```python
from build123d import *

# Parameters (mm, degrees)
SKETCH1_W           = 31
SKETCH1_H           = 15
BOSS_EXTRUDE1_DEPTH = 5
SKETCH2_W           = 15
SKETCH2_H           = 15
BOSS_EXTRUDE2_DEPTH = 3
SKETCH3_W           = 15
SKETCH3_H           = 6
BOSS_EXTRUDE3_DEPTH = 15
SKETCH4_W           = 1
SKETCH4_H           = 6
RIB_DEPTH           = 3
SKETCH5_R           = 4
CUT_EXTRUDE1_DEPTH  = 39.356876828
SKETCH6_R           = 3
CUT_EXTRUDE2_DEPTH  = 7.8
FILLET1_R           = 5
FILLET2_R           = 5
FILLET3_R           = 2


with BuildPart() as part:
    # Sketch1 → Boss-Extrude1 (new body)
    with BuildSketch(Plane(origin=(0, 0, 0), x_dir=(1, 0, 0), z_dir=(0, 1, 0))):
        with Locations((15.5, 7.5)):
            Rectangle(SKETCH1_W, SKETCH1_H)
    extrude(amount=BOSS_EXTRUDE1_DEPTH)

    # Sketch2 → Boss-Extrude2 (add)
    with BuildSketch(Plane(origin=(0, 5, 0), x_dir=(1, 0, 0), z_dir=(0, 1, 0))):
        with Locations((7.5, 7.5)):
            Rectangle(SKETCH2_W, SKETCH2_H)
    extrude(amount=BOSS_EXTRUDE2_DEPTH)

    # Sketch3 → Boss-Extrude3 (add)
    with BuildSketch(Plane(origin=(0, 5, 0), x_dir=(1, 0, 0), z_dir=(0, 1, 0))):
        with Locations((23.5, 7.5)):
            Rectangle(SKETCH3_W, SKETCH3_H)
    extrude(amount=BOSS_EXTRUDE3_DEPTH)

    # Sketch4 → rib (add)
    with BuildSketch(Plane(origin=(0, 5, 0), x_dir=(1, 0, 0), z_dir=(0, 1, 0))):
        with Locations((15.5, 7.5)):
            Rectangle(SKETCH4_W, SKETCH4_H)
    extrude(amount=RIB_DEPTH)

    # Sketch5 → Cut-Extrude1 (cut, through all)
    with BuildSketch(Plane.XY.offset(-4.5)):
        with Locations((23.5, 12.5)):
            Circle(SKETCH5_R)
    extrude(amount=-CUT_EXTRUDE1_DEPTH, mode=Mode.SUBTRACT)

    # Sketch6 → Cut-Extrude2 (cut)
    with BuildSketch(Plane(origin=(0, 8, 0), x_dir=(1, 0, 0), z_dir=(0, 1, 0))):
        with Locations(Location((7.5, 7.5, 0), (0, 0, 270))):
            Circle(SKETCH6_R)
    extrude(amount=-CUT_EXTRUDE2_DEPTH, mode=Mode.SUBTRACT)

    # Fillet1
    fillet1_edges = [part.edges().sort_by_distance(p)[0] for p in [
        (16, 20, -7.5),
        (31, 20, -7.5),
    ]]
    fillet(fillet1_edges, radius=FILLET1_R)

    # Fillet2
    # the kernel refuses this fillet: 5 mm, written as the material it takes off along each edge
    with BuildSketch(Plane(origin=(31, -12.5, -15), x_dir=(0, 0, 1), z_dir=(0, 1, 0))) as fillet2_piece_1:
        with BuildLine():
            CenterArc((FILLET2_R, -FILLET2_R), FILLET2_R, 90, 90)
            Line((0, -FILLET2_R), (0, 0))
            Line((0, 0), (FILLET2_R, 0))
        make_face()
    extrude(amount=30, mode=Mode.SUBTRACT)
    with BuildSketch(Plane(origin=(31, -12.5, 0), x_dir=(0, 0, -1), z_dir=(0, 1, 0))) as fillet2_piece_2:
        with BuildLine():
            CenterArc((FILLET2_R, FILLET2_R), FILLET2_R, 180, 90)
            Line((0, FILLET2_R), (0, 0))
            Line((0, 0), (FILLET2_R, 0))
        make_face()
    extrude(amount=30, mode=Mode.SUBTRACT)
    with BuildSketch(Plane(origin=(15, 5, -15), x_dir=(-1, 0, 0), z_dir=(0, 1, 0))) as fillet2_piece_3:
        with BuildLine():
            CenterArc((4.974937186, 5), FILLET2_R, 185.739170477, 84.260829523)
            Line((0, 4.5), (0, 0))
            Line((0, 0), (4.974937186, 0))
        make_face()
    extrude(amount=15.437342964, mode=Mode.SUBTRACT)
    with BuildSketch(Plane(origin=(15, 5, 0), x_dir=(-1, 0, 0), z_dir=(0, 1, 0))) as fillet2_piece_4:
        with BuildLine():
            CenterArc((4.974937186, -5), FILLET2_R, 90, 84.260829523)
            Line((0, -4.5), (0, 0))
            Line((0, 0), (4.974937186, 0))
        make_face()
    extrude(amount=15.437342964, mode=Mode.SUBTRACT)
    with BuildSketch(Plane(origin=(0, 20.5, 0), x_dir=(1, 0, 0), z_dir=(0, -1, 0))) as fillet2_piece_5:
        with BuildLine():
            CenterArc((FILLET2_R, -FILLET2_R), FILLET2_R, 90, 90)
            Line((0, -FILLET2_R), (0, 0))
            Line((0, 0), (FILLET2_R, 0))
        make_face()
    extrude(amount=33, mode=Mode.SUBTRACT)
    with BuildSketch(Plane(origin=(0, 20.5, -15), x_dir=(1, 0, 0), z_dir=(0, -1, 0))) as fillet2_piece_6:
        with BuildLine():
            CenterArc((FILLET2_R, FILLET2_R), FILLET2_R, 180, 90)
            Line((0, FILLET2_R), (0, 0))
            Line((0, 0), (FILLET2_R, 0))
        make_face()
    extrude(amount=33, mode=Mode.SUBTRACT)

    # Fillet3
    fillet3_edges = [part.edges().sort_by_distance(p)[0] for p in [
        (16, 8, -7.5),
    ]]
    fillet(fillet3_edges, radius=FILLET3_R)


solid = part.part
```
The listing builds one solid part. Answer for the finished solid, in the listing's coordinates (mm). A direction names the side the tool comes from. Coordinates: 2 decimals unless noted, no trailing zeros. Write each loop counter-clockwise with the first axis right and the second up, starting at its lowest first coordinate (ties: lowest second). Pieces come first, ordered by that corner, then holes. Notation, with made-up numbers: (55.5, -32.75) - (83.5, -32.75) arc R19 cw to (83.5, -14.75) - close; hole circle Ø7 at (41, 35). An arc over 180 degrees is marked (long way). Return JSON: item names as keys, results as strings. Group by question number.
1. Straight lines are drawn through the part: L1, parallel to X at y = 4.25, z = -7.5; L2, parallel to Y at x = 23.5, z = -7.5; L3, parallel to Y at x = 2, z = -2. For each, find the intervals that lie inside material, in ascending order.
2. Which of the six approach directions +Z, -Z, +X, -X, +Y, -Y give full straight-line access (tool end or side, diameter ignored) to faces 1 (the cylindrical face through (8.4, 4.15, -4.64)), 2 (the flat face through (23, 5, -2)), 3 (the cylindrical face through (13.42, 6.61, -13.67))?
3. A cutting plane is placed at C-C, the plane z = -7.5. Determine the outline of the cut face in (x, y), plus the area to 3 significant figures.
4. A cutting plane is placed at D-D, the plane x = 7.5. Determine the outline of the cut face in (y, z), plus the area to 3 significant figures.
5. A cutting plane is placed at B-B, the plane y = 12.5. Determine the outline of the cut face in (x, z), plus the area to 3 significant figures.
6. A cutting plane is placed at A-A, the plane x = 23.5. Determine the outline of the cut face in (y, z).
7. Given pin 1 (3 mm diameter, centred on y = 10.5, z = -3.5, fed in from -X); pin 2 (10 mm diameter, centred on x = 25, y = 14, fed in from +Z); pin 3 (6 mm diameter, centred on x = 8.5, z = -11.5, fed in from +Y), each flat-ended and moving along its own axis, determine where each tip first touches the part or whether it passes through.
Ans:
{
 "1": {"L1": "0 to 4.5, 10.5 to 31", "L2": "0 to 8.5, 16.5 to 20", "L3": "0 to 8"},
 "2": {"face 1": "+Y", "face 2": "+Z, +X, +Y", "face 3": "-Z, +X, +Y"},
 "3": {"outline": "(0, 0) - (31, 0) - (31, 15) arc R5 ccw to (26, 20) - (21, 20) arc R5 ccw to (16, 15) - (16, 10) arc R2 cw to (14, 8) - (10.5, 8) - (10.5, 0.2) - (4.5, 0.2) - (4.5, 8) - (0, 8) - close; hole circle Ø8 at (23.5, 12.5)", "area": "321 mm²"},
 "4": {"outline": "(0, -15) - (8, -15) - (8, -10.5) - (0.2, -10.5) - (0.2, -4.5) - (8, -4.5) - (8, 0) - (0, 0) - close", "area": "73.2 mm²"},
 "5": {"outline": "(16, -10.5) - (19.5, -10.5) - (19.5, -4.5) - (16, -4.5) - close; (27.5, -10.5) - (30.97, -10.5) arc R5 ccw to (31, -10) - (31, -5) arc R5 ccw to (30.97, -4.5) - (27.5, -4.5) - close", "area": "42.0 mm²"},
 "6": {"outline": "(0, -15) - (5, -15) - (5, -10.5) - (8.5, -10.5) - (8.5, -4.5) - (5, -4.5) - (5, 0) - (0, 0) - close; (16.5, -10.5) - (20, -10.5) - (20, -4.5) - (16.5, -4.5) - close"},
 "7": {"pin 1": "x = 15.9", "pin 2": "z = -4.5", "pin 3": "y = 8"}
}
